Can you work these out from the model? Positions are in its coordinate system, mm. Round coordinates to 2 decimals unless told otherwise and drop trailing zeros. Write each loop counter-clockwise with the first axis right and the second up, starting at its lowest first coordinate (ties: lowest second). Pieces come first, ordered by that corner, then holes. Notation, with made-up numbers: M 83.25,-25.5 L 99.25,-25.5 A12 cw 99.25,-21.5 Z; hole C 14.25,-17.75 d7. An arc over 180 degrees is marked long. Answer as a JSON object with one key per item and string values. Group by question number.
1) I'm going to push flat-ended pins straight in: pin 1 Ø16 at (x, y) = (0, 13) entering from -Z; pin 2 Ø1 at (x, z) = (36, 1) entering from -Y; pin 3 Ø11 at (x, y) = (11.26, -6.5) entering from +Z; pin 4 Ø1 at (x, z) = (-23.5, 1.5) entering from +Y. Where does each tip first touch, or does it pass through?
2) Suppose I cut it at A-A, the plane y = 13. Write out the boundary of the cut face in (x, z), and give its area (3 significant figures).
3) Suppose I cut it at D-D, the plane z = 1.9. Write out the boundary of the cut face in (x, y), and give its area (3 significant figures).
4) Please list where these lines run through material, in increasing order: L1, parallel to X at y = -12.5, z = 2.2; L2, parallel to Y at x = -3, z = 4.4; L3, parallel to Y at x = -16.5, z = 1.9. Write a range as [from, to].
5) Suppose I cut it at C-C, the plane y = -6.5. Write out the boundary of the cut face in (x, z), and give its area (3 significant figures).
6) Suppose I cut it at B-B, the plane x = 0. Write out the boundary of the cut face in (y, z).
7) If we mould it in two halves opening along Y, with no side actions, what happens to faces 1 (the flat face through (-1, 1, 5)), 2 (the flat face through (0.805, 64.625, 2.465)), 3 (the cylindrical face through (4.265, -6.192, 2.465))? For each: +Y half, -Y half, draft (parallel to the pull), parting line (faces both ways), or undercut.
from build123d import *

# Parameters (mm, degrees)
SKETCH1_W           = 115
SKETCH1_H           = 132.8
SKETCH1_R           = 7
BOSS_EXTRUDE1_DEPTH = 5
CUT_EXTRUDE1_REACH  = 117
CUT_EXTRUDE2_REACH  = 117


with BuildPart() as part:
    # Sketch1 → Boss-Extrude1 (new body)
    with BuildSketch(Plane.XY):
        Rectangle(SKETCH1_W, SKETCH1_H)
        with Locations((0, 13)):
            Circle(SKETCH1_R, mode=Mode.SUBTRACT)
        with Locations((-11.258330249, -6.5)):
            Circle(SKETCH1_R, mode=Mode.SUBTRACT)
        with Locations((11.258330249, -6.5)):
            Circle(SKETCH1_R, mode=Mode.SUBTRACT)
    extrude(amount=BOSS_EXTRUDE1_DEPTH)

    # Sketch2 → Cut-Extrude1 (cut, up to next)
    with BuildSketch(Plane(origin=(57.5, 0, 0), x_dir=(0, 0, -1), z_dir=(1, 0, 0)), mode=Mode.PRIVATE) as cut_extrude1_sk1:
        Polygon((-5, -66.4), (0, -66.4), (0, -59.259259966), align=None)
    cut_extrude1_tool1 = extrude(cut_extrude1_sk1.sketch, amount=-CUT_EXTRUDE1_REACH, mode=Mode.PRIVATE) & part.part
    add(cut_extrude1_tool1.solids().sort_by_distance((57.5, -64.019753, 1.666667))[0], mode=Mode.SUBTRACT)

    # Sketch3 → Cut-Extrude2 (cut, up to next)
    with BuildSketch(Plane(origin=(57.5, 0, 0), x_dir=(0, 0, -1), z_dir=(1, 0, 0)), mode=Mode.PRIVATE) as cut_extrude2_sk1:
        Polygon((-5, 66.4), (0, 66.4), (0, 62.898962309), align=None)
    cut_extrude2_tool1 = extrude(cut_extrude2_sk1.sketch, amount=-CUT_EXTRUDE2_REACH, mode=Mode.PRIVATE) & part.part
    add(cut_extrude2_tool1.solids().sort_by_distance((57.5, 65.232987, 1.666667))[0], mode=Mode.SUBTRACT)


solid = part.part
Results:
{
 "1": {"pin 1": "z = 0", "pin 2": "y = -61.4", "pin 3": "through", "pin 4": "y = 64.3"},
 "2": {"outline": "M -57.5,0 L -7,0 L -7,5 L -57.5,5 Z; M 7,0 L 57.5,0 L 57.5,5 L 7,5 Z", "area": "505 mm^2"},
 "3": {"outline": "M -57.5,-61.97 L 57.5,-61.97 L 57.5,64.23 L -57.5,64.23 Z; hole C -11.26,-6.5 d14; hole C 0,13 d14; hole C 11.26,-6.5 d14", "area": "14,100 mm^2"},
 "4": {"L1": "[-57.5, -14.86], [-7.65, 7.65], [14.86, 57.5]", "L2": "[-65.54, 6.68], [19.32, 65.98]", "L3": "[-61.97, -11.14], [-1.86, 64.23]"},
 "5": {"outline": "M -57.5,0 L -18.26,0 L -18.26,5 L -57.5,5 Z; M -4.26,0 L 4.26,0 L 4.26,5 L -4.26,5 Z; M 18.26,0 L 57.5,0 L 57.5,5 L 18.26,5 Z", "area": "435 mm^2"},
 "6": {"outline": "M -66.4,5 L -59.26,0 L 6,0 L 6,5 Z; M 20,0 L 62.9,0 L 66.4,5 L 20,5 Z"},
 "7": {"face 1": "draft", "face 2": "+Y half", "face 3": "undercut"}
}
